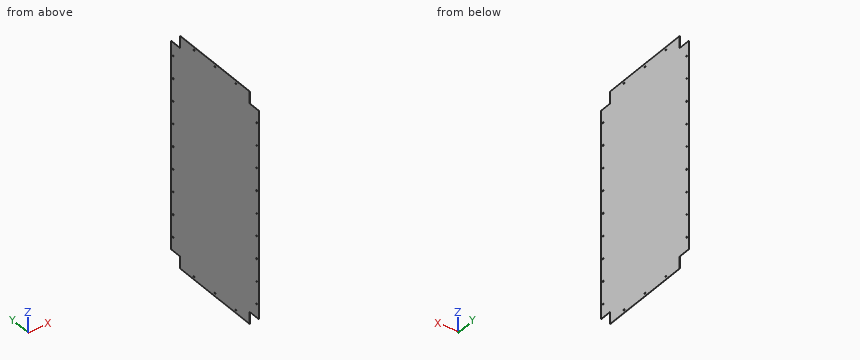
```python
from build123d import *

# Parameters (mm, degrees)
SKETCH1_W               = 1559.92
SKETCH1_H               = 759.96
SKETCH1_R               = 4.1
BOSS_EXTRUDE1_DEPTH     = 1
CUT_EXTRUDE1_DEPTH      = 10
CUT_EXTRUDE1_DEPTH_BACK = 10
SKETCH2_W               = 81
SKETCH2_H               = 81


with BuildPart() as part:
    # Sketch1 → Boss-Extrude1 (new body)
    with BuildSketch(Plane(origin=(0, 0, 0), x_dir=(0, 0, -1), z_dir=(1, 0, 0))):
        Rectangle(SKETCH1_W, SKETCH1_H)
        with Locations((-759.96, 359.98)):
            Circle(SKETCH1_R, mode=Mode.SUBTRACT)
        with Locations((-759.96, -359.98)):
            Circle(SKETCH1_R, mode=Mode.SUBTRACT)
        with Locations((-607.97, 359.98)):
            Circle(SKETCH1_R, mode=Mode.SUBTRACT)
        with Locations((-607.97, -359.98)):
            Circle(SKETCH1_R, mode=Mode.SUBTRACT)
        with Locations((-455.98, 359.98)):
            Circle(SKETCH1_R, mode=Mode.SUBTRACT)
        with Locations((-455.98, -359.98)):
            Circle(SKETCH1_R, mode=Mode.SUBTRACT)
        with Locations((-303.99, 359.98)):
            Circle(SKETCH1_R, mode=Mode.SUBTRACT)
        with Locations((-303.99, -359.98)):
            Circle(SKETCH1_R, mode=Mode.SUBTRACT)
        with Locations((-152, 359.98)):
            Circle(SKETCH1_R, mode=Mode.SUBTRACT)
        with Locations((-152, -359.98)):
            Circle(SKETCH1_R, mode=Mode.SUBTRACT)
        with Locations((-0.01, 359.98)):
            Circle(SKETCH1_R, mode=Mode.SUBTRACT)
        with Locations((-0.01, -359.98)):
            Circle(SKETCH1_R, mode=Mode.SUBTRACT)
        with Locations((151.98, 359.98)):
            Circle(SKETCH1_R, mode=Mode.SUBTRACT)
        with Locations((151.98, -359.98)):
            Circle(SKETCH1_R, mode=Mode.SUBTRACT)
        with Locations((303.97, 359.98)):
            Circle(SKETCH1_R, mode=Mode.SUBTRACT)
        with Locations((303.97, -359.98)):
            Circle(SKETCH1_R, mode=Mode.SUBTRACT)
        with Locations((455.96, 359.98)):
            Circle(SKETCH1_R, mode=Mode.SUBTRACT)
        with Locations((455.96, -359.98)):
            Circle(SKETCH1_R, mode=Mode.SUBTRACT)
        with Locations((607.95, 359.98)):
            Circle(SKETCH1_R, mode=Mode.SUBTRACT)
        with Locations((607.95, -359.98)):
            Circle(SKETCH1_R, mode=Mode.SUBTRACT)
        with Locations((759.94, 359.98)):
            Circle(SKETCH1_R, mode=Mode.SUBTRACT)
        with Locations((759.94, -359.98)):
            Circle(SKETCH1_R, mode=Mode.SUBTRACT)
        with Locations((-759.96, 179.990000139)):
            Circle(SKETCH1_R, mode=Mode.SUBTRACT)
        with Locations((-759.96, 0)):
            Circle(SKETCH1_R, mode=Mode.SUBTRACT)
        with Locations((-759.96, -179.990000139)):
            Circle(SKETCH1_R, mode=Mode.SUBTRACT)
        with Locations((759.96, 0)):
            Circle(SKETCH1_R, mode=Mode.SUBTRACT)
        with Locations((759.96, 179.990000139)):
            Circle(SKETCH1_R, mode=Mode.SUBTRACT)
        with Locations((759.96, -179.990000139)):
            Circle(SKETCH1_R, mode=Mode.SUBTRACT)
    extrude(amount=BOSS_EXTRUDE1_DEPTH)

    # Sketch2 → Cut-Extrude1 (cut, two sides: drawn at the far end of the back side and taken through both)
    with BuildSketch(Plane(origin=(0, 0, 0), x_dir=(0, 0, -1), z_dir=(1, 0, 0)).offset(-CUT_EXTRUDE1_DEPTH_BACK)):
        with Locations((-739.46, 339.48)):
            Rectangle(SKETCH2_W, SKETCH2_H)
        with Locations((-739.46, -339.48)):
            Rectangle(SKETCH2_W, SKETCH2_H)
        with Locations((739.46, -339.48)):
            Rectangle(SKETCH2_W, SKETCH2_H)
        with Locations((739.46, 339.48)):
            Rectangle(SKETCH2_W, SKETCH2_H)
    extrude(amount=CUT_EXTRUDE1_DEPTH + CUT_EXTRUDE1_DEPTH_BACK, mode=Mode.SUBTRACT)


solid = part.part
```
CAD build for the part. Positions are in the model's coordinates, mm. Round coordinates to 2 decimals unless told otherwise and drop trailing zeros. Order: outer loops, then holes, each group sorted by start corner. A loop starts at its lowest first (then second) coordinate and runs counter-clockwise, first axis right, second up. Notation, with made-up numbers: (-5, -24.5) -> (10, -24.5) arc R9 cw to (10, -19.5) -> close; hole circle Ø8 at (60.25, 89). An arc over 180 degrees is marked (long way). One line per question, with ' | ' between items.
Q1. Slice it at A-A (x = 0.3). Give the number of separate pieces and of enclosed holes in the cut face, then the cut area to 3 significant figures.
Completed:
separate pieces: 1 | enclosed holes: 24 | area: 1,160,000 mm^2
Q2. Probe probe 1 along Y at (x, z) = (0.4, 303.99); probe 2 along Y at (x, z) = (0.55, -759.96); probe 3 along Y at (x, z) = (0.7, -151). List the from-to ranges inside material, lowest first.
Completed:
probe 1: y = -379.98 to -364.08, -355.88 to 355.88, 364.08 to 379.98 | probe 2: y = -298.98 to -184.09, -175.89 to -4.1, 4.1 to 175.89, 184.09 to 298.98 | probe 3: y = -379.98 to -363.96, -356 to 356, 363.96 to 379.98
Q3. Slice it at B-B (y = -331.5). Write the cut outline in (x, z), then the cut area to 3 significant figures.
Completed:
outline: (0, -698.96) -> (1, -698.96) -> (1, 698.96) -> (0, 698.96) -> close | area: 1,400 mm^2
